Autodesk Inventor part; units mm, degrees
ref_plane "YZ Plane" through (0, 0, 0) normal (1, 0, 0) x (0, 1, 0)
ref_plane "XZ Plane" through (0, 0, 0) normal (0, 1, 0) x (-1, 0, 0)
ref_plane "XY Plane" through (0, 0, 0) normal (0, 0, 1) x (1, 0, 0)
sketch "スケッチ1" plane through (0, 0, 0) normal (0, 1, 0) x (-1, 0, 0)
  line L0 (130, 81) -> (-130, 81)
  line L1 (-130, 81) -> (-130, -81)
  line L2 (-130, -81) -> (130, -81)
  line L3 (130, -81) -> (130, 81)
  line L4 (130, 81) -> (-130, -81) construction
  line L5 (-130, 81) -> (130, -81) construction
  point P0 (0, 0)
  dimension "d0" = 260
  dimension "d1" = 162
extrude "押し出し1" add sketch "スケッチ1" along normal blind 3
sketch "スケッチ7" plane through (0, 3, 0) normal (0, 1, 0) x (1, 0, 0)
  line L0 (-130, 81) -> (-130, -81)
  line L1 (130, -81) -> (130, 81)
  line L2 (130, 81) -> (-130, 81)
  point P0 (0, 0)
  point P1 (-116, 67)
  point P2 (112, 67)
  point P3 (112, -63)
  point P4 (-116, -63)
  dimension "d23" = 14
  dimension "d25" = 130
  dimension "d26" = 130
  dimension "d27" = 14
  dimension "d29" = 14
  dimension "d38" = 228
  dimension "d39" = 228
  dimension "d40" = 14
hole "穴1" at (-116, 3, -67) at (112, 3, -67) at (112, 3, 63) at (-116, 3, 63) direction (0, -1, 0) diameter 3.2 depth 8
sketch "スケッチ8" plane through (0, 3, 0) normal (0, 1, 0) x (1, 0, 0)
  line L0 (130, 81) -> (-130, 81)
  line L1 (-130, 81) -> (126, 81)
  line L2 (126, 81) -> (126, -77)
  line L3 (126, -77) -> (-130, -77)
  line L4 (-130, -77) -> (-130, 81)
  circle A0 centre (-116, 67) radius 1.6
  circle A1 centre (112, 67) radius 1.6
  circle A2 centre (-116, -63) radius 1.6
  circle A3 centre (-116, -63) radius 1.6
  circle A4 centre (112, -63) radius 1.6
  circle A5 centre (112, 67) radius 1.6
  circle A6 centre (-116, 67) radius 1.6
  line L5 (130, -81) -> (130, 81)
  line L6 (130, 81) -> (-130, 81)
  line L7 (-130, 81) -> (-130, -81)
  line L8 (-130, -81) -> (130, -81)
  point P0 (0, 0)
  dimension "d41" = 14
  dimension "d42" = 14
  dimension "d43" = 14
extrude "押し出し4" cut sketch "スケッチ8" against normal blind 10 contours L5 L8 L7 L3 L2 L0
fillet "フィレット1" radius 5 4 edges at (-130, 1.5, -81) (-130, 1.5, 77) (126, 1.5, -81) (126, 1.5, 77)
sketch "スケッチ9" plane through (0, 3, 0) normal (0, 1, 0) x (1, 0, 0)
  line L0 (-130, 76) -> (-130, -72)
  line L1 (-89.9, 81) -> (-69.9, 81)
  line L2 (-69.8, 81) -> (-49.8, 81)
  line L3 (-49.7, 81) -> (-29.7, 81)
  line L4 (-29.7, -77) -> (-49.7, -77)
  line L5 (0, 0) -> (0, 16.1014)
  circle A0 centre (-116, 67) radius 1.6
  line L6 (126, -72) -> (126, 76)
  line L7 (121, 81) -> (-125, 81)
  line L8 (-125, -77) -> (121, -77)
  line L9 (-69.8, 81) -> (-49.8, 81)
  line L10 (-49.8, 81) -> (-49.8, -77)
  line L11 (-49.8, -77) -> (-69.8, -77)
  line L12 (-69.8, -77) -> (-69.8, 81)
  line L13 (45.8, 81) -> (65.8, 81)
  line L14 (65.8, 81) -> (65.8, -77)
  line L15 (65.8, -77) -> (45.8, -77)
  line L16 (45.8, -77) -> (45.8, 81)
  line L17 (-69.9, 81) -> (-89.9, 81)
  line L18 (-89.9, 81) -> (-89.9, -77)
  line L19 (-89.9, -77) -> (-69.9, -77)
  line L20 (-69.9, -77) -> (-69.9, 81)
  line L21 (121, 81) -> (-125, 81)
  line L22 (-49.7, 81) -> (-29.7, 81)
  line L23 (-29.7, 81) -> (-29.7, -77)
  line L24 (-29.7, -77) -> (-49.7, -77)
  line L25 (-49.7, -77) -> (-49.7, 81)
  point P0 (-79.9, 61)
  point P1 (-39.7, 61)
  point P2 (-79.9, -57)
  point P3 (-39.7, -57)
  point P4 (75.9, 61)
  point P5 (35.7, 61)
  point P6 (75.9, -57)
  point P7 (35.7, -57)
  point P8 (-79.9, 81)
  point P9 (-59.8, 61)
  point P10 (55.8, 61)
  point P11 (55.8, -57)
  point P12 (-59.8, -57)
  dimension "d77" = 118
  dimension "d114" = 20
  dimension "d115" = 20
  dimension "d116" = 20
  dimension "d117" = 20
  dimension "d118" = 20
  dimension "d119" = 20
  dimension "d120" = 20
  dimension "d121" = 20
  dimension "d122" = 70.2
  dimension "d123" = 70.2
  dimension "d124" = 20
  dimension "d125" = 70.2
  dimension "d126" = 70.2
  dimension "d127" = 10
  dimension "d128" = 10
  dimension "d129" = 10
  dimension "d130" = 10
  dimension "d131" = 10
  dimension "d132" = 0.1
  dimension "d133" = 50.1
  dimension "d134" = 50.1
  dimension "d135" = 10
  dimension "d136" = 118
  dimension "d137" = 50.1
  dimension "d138" = 10
  dimension "d139" = 0.1
  dimension "d140" = 10
  dimension "d141" = 90.3
  dimension "d142" = 90.3
  dimension "d143" = 90.3
  dimension "d144" = 90.3
  dimension "d145" = 50.1
hole "穴2" at (-79.9, 3, -61) at (-39.7, 3, -61) at (-79.9, 3, 57) at (-39.7, 3, 57) at (35.7, 3, 57) at (75.9, 3, 57) at (35.7, 3, -61) at (75.9, 3, -61) direction (0, -1, 0) diameter 3.2 depth 8
sketch "スケッチ12" plane through (0, 0, 0) normal (0, -1, 0) x (1, 0, 0)
  circle A0 centre (75.9, -61) radius 1.6
  circle A1 centre (35.7, -61) radius 1.6
  circle A2 centre (75.9, 57) radius 1.6
  circle A3 centre (35.7, 57) radius 1.6
  circle A4 centre (-39.7, 57) radius 1.6
  circle A5 centre (-79.9, 57) radius 1.6
  circle A6 centre (-39.7, -61) radius 1.6
  circle A7 centre (-79.9, -61) radius 1.6
  arc A8 (126, 72) -> (121, 77) centre (121, 72) ccw
  line L0 (121, 77) -> (-125, 77)
  arc A9 (-125, 77) -> (-130, 72) centre (-125, 72) ccw
  line L1 (-130, -76) -> (-130, 72)
  arc A10 (-130, -76) -> (-125, -81) centre (-125, -76) ccw
  line L2 (121, -81) -> (-125, -81)
  arc A11 (121, -81) -> (126, -76) centre (121, -76) ccw
  line L3 (126, -76) -> (126, 72)
  circle A12 centre (-116, 63) radius 1.6
  circle A13 centre (112, 63) radius 1.6
  circle A14 centre (112, -67) radius 1.6
  circle A15 centre (-116, -67) radius 1.6
  circle A16 centre (-116, 63) radius 3
  circle A17 centre (-116, -67) radius 3
  circle A18 centre (112, -67) radius 3
  circle A19 centre (112, 63) radius 3
  point P0 (0, 0)
  dimension "d108" = 6
  dimension "d109" = 6
  dimension "d110" = 6
  dimension "d111" = 6
  dimension "d14" = 30
  dimension "d15" = 30
  dimension "d16" = 30
  dimension "d17" = 30
extrude "押し出し6" cut sketch "スケッチ12" against normal blind 2 contours A12 | A13 | A14 | A15 | A16 | A17 | A18 | A19
equation "\"d42\" = d41"
equation "\"d43\" = d41"
equation "\"d139\" = d132"
equation "\"d109\" = d108"
equation "\"d110\" = d109"
equation "\"d111\" = d108"
properties part number "BP_BOX-Under" material "アセタール樹脂、白"
Here's how the part is built. I have some questions about the finished solid (model axes, mm). A direction names the side the tool comes from. Round coordinates to 2 decimals unless told otherwise and drop trailing zeros. Answer as CSV lines item,"result". Start each with the question number.
1. Thinking about a two-plate mould opening in Z: for faces 1 (the cylindrical face through (-113.14, 0.99, 63.9)), 2 (the cylindrical face through (125, 1, 75)), 3 (the cylindrical face through (124, 1, -80)), which applies, released by +Z, released by -Z, zero draft, split by the parting line, or undercut?
2. I need wall thicknesses on probe 1 along X at (y, z) = (1.6, -61); probe 2 along Z at (x, y) = (112, 0.6); probe 3 along Z at (x, y) = (-116, 2.8). Which ranges of each line are inside material? Lowest first, please.
3. On a 3-axis mill with a long thin cutter (end or side, diameter ignored), from which of +Z, -Z, +X, -X, +Y, -Y can I reach the whole of each face in a straight line? I mean faces 4 (the flat face through (113.3, 2, 61.7)), 5 (the cylindrical face through (-128, 1, 76)). Say none if no direction works.
4. I'm going to push flat-ended pins straight in: pin 1 Ø2.5 at (x, z) = (112, 63) entering from -Y; pin 2 Ø1.8 at (x, z) = (111, 62) entering from -Y. Where does each tip first touch, or does it pass through?
Check result:
1,face 1,"undercut"
1,face 2,"released by +Z"
1,face 3,"released by -Z"
2,probe 1,"x = -130 to -81.5, -78.3 to -41.3, -38.1 to 34.1, 37.3 to 74.3, 77.5 to 126"
2,probe 2,"z = -81 to -70, -64 to 60, 66 to 77"
2,probe 3,"z = -81 to -68.6, -65.4 to 61.4, 64.6 to 77"
3,face 4,"-Y"
3,face 5,"+Z, -X, +Y, -Y"
4,pin 1,"passes through"
4,pin 2,"stops at y = 2"
